Part model, mm, in its own coordinate system. A direction names the side the tool comes from. Round coordinates to 2 decimals unless told otherwise and drop trailing zeros. Write each loop counter-clockwise with the first axis right and the second up, starting at its lowest first coordinate (ties: lowest second). Pieces come first, ordered by that corner, then holes.
1) Drill centre lines: L1, parallel to Z at x = -0.5, y = -290.5 (3 decimals); L2, parallel to X at y = -267, z = 0.25 (3 decimals). Where is each one in solid material? Low to high.
2) Which spindle directions (+Z, -Z, +X, -X, +Y, -Y) get a long thin tool onto all of the face, cutting with end or side? Do faces 1 (the flat face through (-19.05, -150, 9)), 2 (the flat face through (-10, -150, 22.225)). Say none if no direction does.
3) Saw through at B-B on y = -103.5. Write the cut outline in (x, z) (3 decimals).
4) Pull direction Y, two halves, no side cores. Call faces 3 (the flat face through (-21, 0, 10)), 4 (the flat face through (3.175, -150, 9)), 5 (the cylindrical face through (-20.66, -288.93, 9.8)): +Y half, -Y half, draft (parallel to the pull), parting line (faces both ways), or undercut.
5) Saw through at A-A on x = -9. Write the cut outline in (y, z) (3 decimals).
```python
from build123d import *

# Parameters (mm, degrees)
F0_W     = 25.4
F0_H     = 25.4
F0_W_2   = 19.05
F0_H_2   = 19.05
F1_DEPTH = 304.8
F3_D     = 12.7


# Not quite as in the source:
# - a feature names something its author has since deleted; it is built from what else it names


with BuildPart() as f1:
    # F0 (on Front) → F1 (new body)
    with BuildSketch(Plane.XZ):
        with Locations((-9.525, 9.525)):
            Rectangle(F0_W, F0_H)
        with Locations((-9.525, 9.525)):
            Rectangle(F0_W_2, F0_H_2, mode=Mode.SUBTRACT)
    extrude(amount=F1_DEPTH)

    # F3 (through all)
    with Locations(Plane.YZ.offset(3.175)):
        with Locations((-295.275, 9.525)):
            Hole(F3_D / 2)


solid = f1.part
```
Completed:
1. L1: z = -3.175 to 0, 19.05 to 22.225
1. L2: x = -22.225 to -19.05, 0 to 3.175
2. face 1: +Y, -Y
2. face 2: +Z, +X, -X, +Y, -Y
3. outline: (-22.225, -3.175) - (3.175, -3.175) - (3.175, 22.225) - (-22.225, 22.225) - close; hole (-19.05, 0) - (0, 0) - (0, 19.05) - (-19.05, 19.05) - close
4. face 3: +Y half
4. face 4: draft
4. face 5: undercut
5. outline: (-304.8, -3.175) - (0, -3.175) - (0, 0) - (-304.8, 0) - close; (-304.8, 19.05) - (0, 19.05) - (0, 22.225) - (-304.8, 22.225) - close
